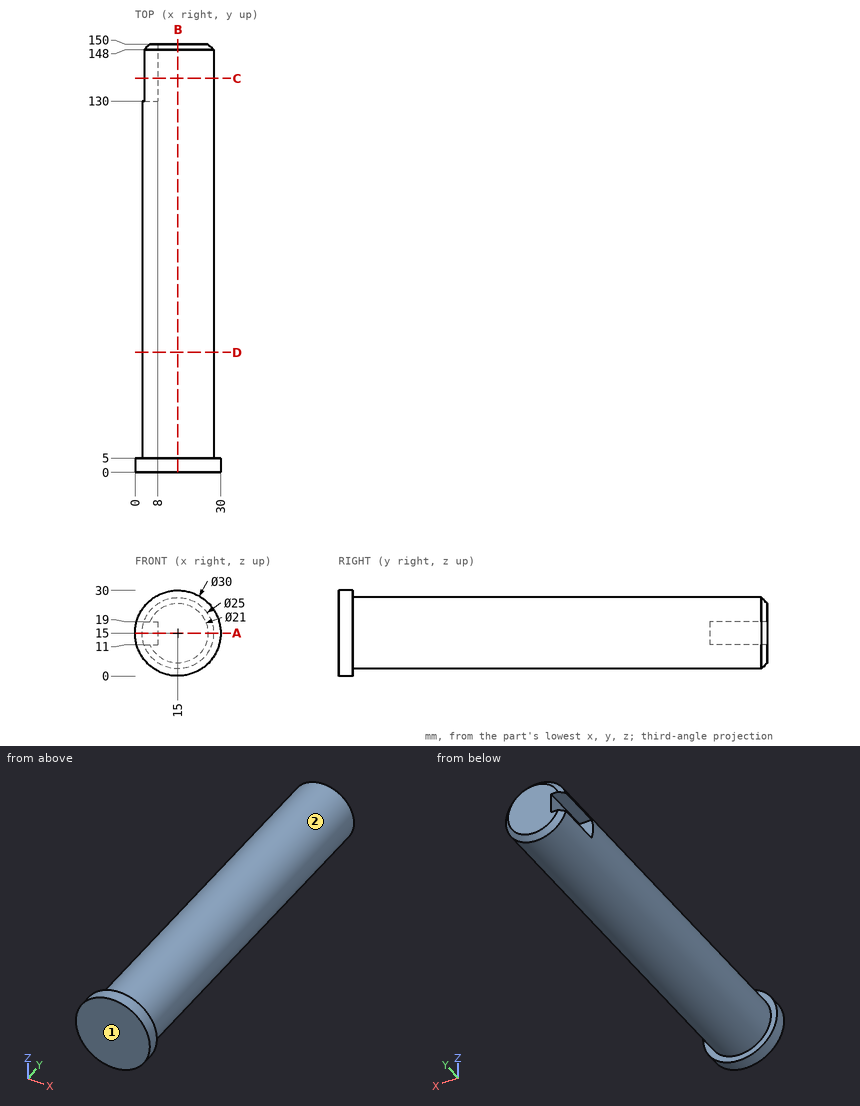
Geometry: see drawing. Coordinates: mm, zero at the bounding-box minimum. A direction names the side the tool comes from. Coordinates: 2 decimals unless noted, no trailing zeros. Order: outer loops, then holes, each group sorted by start corner. A loop starts at its lowest first (then second) coordinate and runs counter-clockwise, first axis right, second up. Notation, with made-up numbers: (37, 8.25) - (78, 8.25) arc R18 cw to (78, 23.25) - close; hole circle Ø3 at (41, 48). An arc over 180 degrees is marked (long way). Write each question's results on one line, items separated by ' | '.
(1) First-contact query: pin 1 Ø1.5 at (y, z) = (67.5, 15.5) entering from -X; pin 2 Ø1.6 at (x, z) = (4.5, 16) entering from +Y; pin 3 Ø2 at (x, y) = (16, 103) entering from -Z. Flat tips, straight axial feed; report the tip coordinate or a pass-through.
Values found:
pin 1: stops at x = 2.5 | pin 2: stops at y = 130 | pin 3: stops at z = 2.5
(2) Section query D-D, the plane y = 42. Return the cut outline in (x, z).
Values found:
outline: circle Ø25 at (15, 15)
(3) Line query: line 1 (Z direction, x = 15, y = 37.5); line 2 (Z direction, x = 5.5, y = 139); line 3 (Y direction, x = 24.5, z = 10.5). Output: solid intervals per line, ascending. Write a range as [from, to].
Values found:
line 1: z = [2.5, 27.5] | line 2: z = [6.88, 11], [19, 23.12] | line 3: y = [0, 149.99]
(4) Set-up query: the marked faces 1 and 2. Return all of +Z, -Z, +X, -X, +Y, -Y with unobstructed straight access to the full face (end or side cutting, diameter ignored); none if empty.
Values found:
face 1: +Z, -Z, +X, -X, -Y | face 2: +Y
(5) Section query A-A, the plane z = 15. Return the cut outline in (x, y), plus the area to 3 significant figures.
Values found:
outline: (0, 0) - (30, 0) - (30, 5) - (27.5, 5) - (27.5, 148) - (25.5, 150) - (8, 150) - (8, 130) - (2.5, 130) - (2.5, 5) - (0, 5) - close | area: 3,660 mm²
(6) Section query B-B, the plane x = 15. Return the cut outline in (y, z).
Values found:
outline: (0, 0) - (5, 0) - (5, 2.5) - (148, 2.5) - (150, 4.5) - (150, 25.5) - (148, 27.5) - (5, 27.5) - (5, 30) - (0, 30) - close
(7) Section query C-C, the plane y = 138. Return the cut outline in (x, z), plus the area to 3 significant figures.
Values found:
outline: (3.16, 11) arc R12.5 ccw (long way) to (3.16, 19) - (8, 19) - (8, 11) - close | area: 449 mm²
